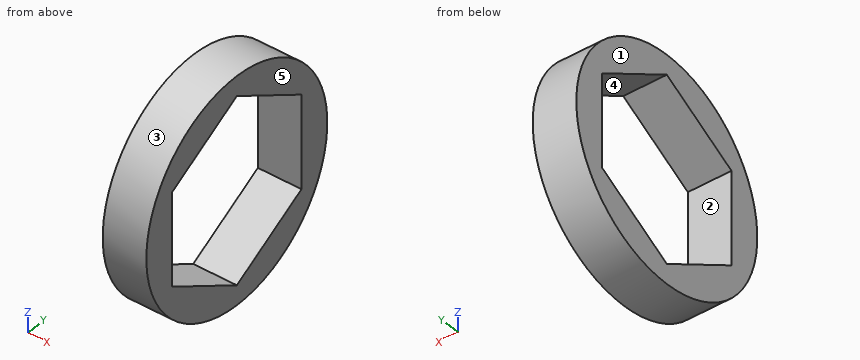
from build123d import *

# Parameters (mm, degrees)
F0_W     = 4
F0_H     = 1.8
F3_DEPTH = 4


with BuildPart() as f1:
    # F0 (on Front) → F1 (revolve)
    with BuildSketch(Plane.XZ):
        with Locations((-19.3521137871, 22.5742971626)):
            Rectangle(F0_W, F0_H)
    revolve(axis=Axis((-20.6097164191, 0, 13.1742971626), (1, 0, 0)))

    # F2 (on face) → F3 (join)
    with BuildSketch(Plane.YZ.offset(-17.3521137871)):
        with BuildLine():
            Line((-7.3612159322, 17.4242971626), (0, 21.6742971626))
            ThreePointArc((0, 21.6742971626), (-4.25, 20.5355130948), (-7.3612159322, 17.4242971626))
        make_face()
        with BuildLine():
            Line((-7.3612159322, 8.9242971626), (-7.3612159322, 17.4242971626))
            ThreePointArc((-7.3612159322, 17.4242971626), (-8.5, 13.1742971626), (-7.3612159322, 8.9242971626))
        make_face()
        with BuildLine():
            Line((0, 4.6742971626), (-7.3612159322, 8.9242971626))
            ThreePointArc((-7.3612159322, 8.9242971626), (-4.25, 5.8130812304), (0, 4.6742971626))
        make_face()
        with BuildLine():
            ThreePointArc((0, 4.6742971626), (4.25, 5.8130812304), (7.3612159322, 8.9242971626))
            Line((7.3612159322, 8.9242971626), (0, 4.6742971626))
        make_face()
        with BuildLine():
            ThreePointArc((8.5, 13.1742971626), (8.2103695235, 15.374259046), (7.3612159322, 17.4242971626))
            Line((7.3612159322, 17.4242971626), (7.3612159322, 8.9242971626))
            ThreePointArc((7.3612159322, 8.9242971626), (8.2103695235, 10.9743352792), (8.5, 13.1742971626))
        make_face()
        with BuildLine():
            ThreePointArc((7.3612159322, 17.4242971626), (4.25, 20.5355130948), (0, 21.6742971626))
            Line((0, 21.6742971626), (7.3612159322, 17.4242971626))
        make_face()
    extrude(amount=-F3_DEPTH)


solid = f1.part
Model file for the job. Use its own axes, mm. Face numbers are marked on the shaded views. A direction names the side the tool comes from. Give positions to 0.01 mm unless a question says otherwise; leave off trailing zeros. Order: outer loops, then holes, each group sorted by start corner. A loop starts at its lowest first (then second) coordinate and runs counter-clockwise, first axis right, second up. Notation, with made-up numbers: M 22.25,52 L 81.25,52 A27 ccw 81.25,84 Z; hole C 81,-38 d1. An arc over 180 degrees is marked long. Put each result on its own line as item: value. Start each with the question number.
(1) Drill centre lines: L1, parallel to Y at x = -20.45, z = 13; L2, parallel to Z at x = -18.45, y = -4; L3, parallel to Y at x = -20.15, z = 16. Where is each one in solid material? Low to high. Write a range as [from, to].
(2) Band-saw the part on C-C on z = 20. Give the cut face in (x, y), then the cut area to 3 significant figures.
(3) Tool access for the marked faces 1 and 2: list every direction of +Z, -Z, +X, -X, +Y, -Y with a clear straight run to the whole face (end or side of a thin tool).
(4) Pull direction Z, two halves, no side cores. Call the marked faces 3, 4 and 5: released by +Z, released by -Z, zero draft, split by the parting line, or undercut.
(5) Pin check, flat tip, straight feed: pin 1 Ø1 at (x, y) = (-19.5, 2) entering from +Z. Stop position of the tip, or through.
(6) Band-saw the part on B-B on y = 2.75. Give the cut face in (x, z), then the cut area to 3 significant figures.
(7) Band-saw the part on A-A on x = -19.15. Give the cut face in (y, z).
Results below:
1. L1: y = [-10.3, -7.36], [7.36, 10.3]
1. L2: z = [3.68, 6.98], [19.36, 22.67]
1. L3: y = [-9.9, -7.36], [7.36, 9.9]
2. outline: M -21.35,-7.71 L -17.35,-7.71 L -17.35,-2.9 L -21.35,-2.9 Z; M -21.35,2.9 L -17.35,2.9 L -17.35,7.71 L -21.35,7.71 Z
2. area: 38.5 mm2
3. face 1: +Z, -Z, -X, +Y, -Y
3. face 2: +X, -X
4. face 3: split by the parting line
4. face 4: undercut
4. face 5: zero draft
5. pin 1: stops at z = 23.36
6. outline: M -21.35,3.25 L -17.35,3.25 L -17.35,6.26 L -21.35,6.26 Z; M -21.35,20.09 L -17.35,20.09 L -17.35,23.1 L -21.35,23.1 Z
6. area: 24.1 mm2
7. outline: C 0,13.17 d20.6; hole M -7.36,8.92 L 0,4.67 L 7.36,8.92 L 7.36,17.42 L 0,21.67 L -7.36,17.42 Z
